Here's how the part is built. I have some questions about the finished solid (model axes, mm). A direction names the side the tool comes from. Give positions to 0.01 mm unless a question says otherwise; leave off trailing zeros. Loops run counter-clockwise (first coordinate to the right, second up) from the corner with the lowest first, then second, coordinate; pieces in that order, holes last. Notation, with made-up numbers: (65.25, 61.25) -> (97.25, 61.25) arc R17 ccw to (97.25, 93.25) -> close; hole circle Ø11 at (65.25, 77). An arc over 180 degrees is marked (long way). Answer in a Markdown table with one row per item. Add a question column.
Item 1: If we section it at D-D (y = 55): Write out the boundary of the cut face in (x, z).
Item 2: If I drill on line 1 (Z direction, x = -19, y = 0); line 2 (X direction, y = -35, z = 51.5); line 3 (Y direction, x = -171, z = 37.5), over which ranges is the centre line in solid material (lowest first)?
Item 3: We'd pull the mould along Z, two halves only. Please class faces 1 (the face through (-135, -31.75, 23)), 2 (the face through (-154, -38, 38.1)), 3 (the face through (-19, 0, 38.1)), 4 (the face through (-304.8, -1, 44)): released by +Z, released by -Z, zero draft, split by the parting line, or undercut.
Item 4: If we section it at B-B (x = -266): Write out the boundary of the cut face in (y, z).
Item 5: Which directions (+Z, -Z, +X, -X, +Y, -Y) give clear straight access to the entire face, cutting with the end or side of a thin tool? Please do faces 5 (the face through (-18.783, -34.173, 70.852)), 6 (the face through (-19, 55, 50.8)), 7 (the face through (-18.8, 0.3, 101.6)), 8 (the face through (-297.556, -0.889, 94.556)), 9 (the face through (-135, -22, 29.21)).
Item 6: If we section it at C-C (z = 76.2): Write out the boundary of the cut face in (x, y), then the cut area to 3 significant figures.
Item 7: If we section it at A-A (y = 0): Write out the boundary of the cut face in (x, z).
Item 8: For P1, Ø9.5, axis at x = -192, y = -18.5, coming from the +Z side; P2, Ø5, axis at x = -21, y = 59.5, coming from the +Z side, each with a flat end and sliding along its axis, tell me the tip position at first contact or that it passes through.
```python
from build123d import *

# Parameters (mm, degrees)
F1_DEPTH = 63.5
F2_SIZE  = 14.2875
F3_R     = 12.7
F4_DEPTH = 38.1
F5_DEPTH = 273.05


with BuildPart() as f1:
    # F0 (on Front) → F1 (new body, symmetric)
    with BuildSketch(Plane.XZ):
        Polygon((-304.8, 0), (0, 0), (0, 50.8), (-38.1, 50.8), (-38.1, 38.1), (-273.05, 38.1), (-273.05, 101.6), (-304.8, 101.6), align=None)
    extrude(amount=F1_DEPTH, both=True)

    # F2
    f2_edges = [f1.edges().sort_by_distance(p)[0] for p in [
        (-304.8, 0, 101.6),
    ]]
    chamfer(f2_edges, length=F2_SIZE)

    # F3 (on Right) → F4 (join)
    with BuildSketch(Plane.YZ):
        with BuildLine():
            Line((-21.093426, 90.350173), (-47.625, 50.8))
            Line((-47.625, 50.8), (47.625, 50.8))
            Line((47.625, 50.8), (21.093426, 90.350173))
            ThreePointArc((21.093426, 90.350173), (0, 101.6), (-21.093426, 90.350173))
        make_face()
        with Locations((0, 76.2)):
            Circle(F3_R, mode=Mode.SUBTRACT)
    extrude(amount=-F4_DEPTH)

    # F3 (on Right) → F5 (cut)
    with BuildSketch(Plane.YZ):
        Polygon((-12.7, 16.51), (-12.7, 0), (12.7, 0), (12.7, 16.51), (31.75, 16.51), (31.75, 29.21), (12.7, 29.21), (12.7, 38.1), (-12.7, 38.1), (-12.7, 29.21), (-31.75, 29.21), (-31.75, 16.51), align=None)
    extrude(amount=-F5_DEPTH, mode=Mode.SUBTRACT)


solid = f1.part
```
Recorded:
| question | item | result |
|---|---|---|
| 1 | outline | (-304.8, 0) -> (0, 0) -> (0, 50.8) -> (-38.1, 50.8) -> (-38.1, 38.1) -> (-273.05, 38.1) -> (-273.05, 101.6) -> (-290.51, 101.6) -> (-304.8, 87.31) -> close |
| 2 | line 1 | z = 38.1 to 63.5, 88.9 to 101.6 |
| 2 | line 2 | x = -304.8 to -273.05, -38.1 to 0 |
| 2 | line 3 | y = -63.5 to -12.7, 12.7 to 63.5 |
| 3 | face 1 | undercut |
| 3 | face 2 | released by +Z |
| 3 | face 3 | released by -Z |
| 3 | face 4 | zero draft |
| 4 | outline | (-63.5, 0) -> (-12.7, 0) -> (-12.7, 16.51) -> (-31.75, 16.51) -> (-31.75, 29.21) -> (-12.7, 29.21) -> (-12.7, 38.1) -> (-63.5, 38.1) -> close; (12.7, 0) -> (63.5, 0) -> (63.5, 38.1) -> (12.7, 38.1) -> (12.7, 29.21) -> (31.75, 29.21) -> (31.75, 16.51) -> (12.7, 16.51) -> close |
| 5 | face 5 | +Z, +X, -Y |
| 5 | face 6 | +Z, +X, +Y |
| 5 | face 7 | +Z, +X |
| 5 | face 8 | +Z, -X, +Y, -Y |
| 5 | face 9 | +X |
| 6 | outline | (-304.8, -63.5) -> (-273.05, -63.5) -> (-273.05, 63.5) -> (-304.8, 63.5) -> close; (-38.1, -30.59) -> (0, -30.59) -> (0, -12.7) -> (-38.1, -12.7) -> close; (-38.1, 12.7) -> (0, 12.7) -> (0, 30.59) -> (-38.1, 30.59) -> close |
| 6 | area | 5,400 mm^2 |
| 7 | outline | (-304.8, 0) -> (-273.05, 0) -> (-273.05, 101.6) -> (-290.51, 101.6) -> (-304.8, 87.31) -> close; (-38.1, 38.1) -> (0, 38.1) -> (0, 63.5) -> (-38.1, 63.5) -> close; (-38.1, 88.9) -> (0, 88.9) -> (0, 101.6) -> (-38.1, 101.6) -> close |
| 8 | P1 | stops at z = 38.1 |
| 8 | P2 | stops at z = 50.8 |
